```python
from build123d import *

# Parameters (mm, degrees)
F0_R     = 27
F1_DEPTH = 3
F2_R     = 27
F2_R_2   = 24
F3_DEPTH = 24
F4_R     = 1
F5_R     = 0.3


with BuildPart() as f1:
    # F0 (on Front) → F1 (new body)
    with BuildSketch(Plane.XZ):
        Circle(F0_R)
    extrude(amount=F1_DEPTH)

    # F2 (on face) → F3 (join)
    with BuildSketch(Plane(origin=(0, 0, 0), x_dir=(-1, 0, 0), z_dir=(0, 1, 0))):
        Circle(F2_R)
        Circle(F2_R_2, mode=Mode.SUBTRACT)
    extrude(amount=F3_DEPTH)

    # F4
    f4_edges = [f1.edges().sort_by_distance(p)[0] for p in [
        (-27, -3, 0),
    ]]
    fillet(f4_edges, radius=F4_R)

    # F5
    f5_edges = [f1.edges().sort_by_distance(p)[0] for p in [
        (27, 24, 0),
        (24, 24, 0),
    ]]
    fillet(f5_edges, radius=F5_R)


solid = f1.part
```
The listing builds one solid part. Answer for the finished solid, in the listing's coordinates (mm). Give positions to 0.01 mm unless a question says otherwise; leave off trailing zeros. Order: outer loops, then holes, each group sorted by start corner. A loop starts at its lowest first (then second) coordinate and runs counter-clockwise, first axis right, second up. Notation, with made-up numbers: (-14.75, 59.5) - (-1.75, 59.5) arc R35 ccw to (-1.75, 97.5) - close; hole circle Ø2 at (36.25, -33). An arc over 180 degrees is marked (long way). Use one line per item in the form item = value. Start each with the question number.
(1) A cutting plane is placed at A-A, the plane x = 0. Write down the section's boundary in (y, z).
(2) Consider line 1 (Z direction, x = 0, y = 6.25); line 2 (Y direction, x = 2, z = 7); line 3 (Z direction, x = -9, y = 18.75). Determine where each line is inside the solid, lowest interval first. Write a range as from..to.
(3) A cutting plane is placed at B-B, the plane y = 5.25. Write down the section's boundary in (x, z), then the cut area to 3 significant figures.
(4) The mould has two halves that part along X. Classify faces 1 (the flat face through (-6, 24, -24)), 2 (the cylindrical face through (23.977, 11.684, 1.055)), 3 (the flat face through (0, 0, 0)): released by +X, released by -X, zero draft, split by the parting line, or undercut.
(5) A cutting plane is placed at C-C, the plane z = 0. Write down the section's boundary in (x, y), then the cut area to 3 significant figures.
(6) Flat-ended cylindrical pins translate along their axes: pin 1 Ø12 at (x, z) = (-5.5, -1) entering from +Y; pin 2 Ø4 at (x, y) = (-8.5, 1.5) entering from -Z; pin 3 Ø3 at (y, z) = (16.5, 2.5) entering from +X. Find the tip coordinate at first contact, or state that the pin passes through.
Ans:
q1.outline = (-3, -26) arc R1 ccw to (-2, -27) - (23.7, -27) arc R0.3 ccw to (24, -26.7) - (24, -24.3) arc R0.3 ccw to (23.7, -24) - (0, -24) - (0, 24) - (23.7, 24) arc R0.3 ccw to (24, 24.3) - (24, 26.7) arc R0.3 ccw to (23.7, 27) - (-2, 27) arc R1 ccw to (-3, 26) - close
q2.line_1 = -27..-24, 24..27
q2.line_2 = -3..0
q2.line_3 = -25.46..-22.25, 22.25..25.46
q3.outline = circle Ø54 at (0, 0); hole circle Ø48 at (0, 0)
q3.area = 481 mm^2
q4.face_1 = zero draft
q4.face_2 = undercut
q4.face_3 = undercut
q5.outline = (-27, -2) arc R1 ccw to (-26, -3) - (26, -3) arc R1 ccw to (27, -2) - (27, 23.7) arc R0.3 ccw to (26.7, 24) - (24.3, 24) arc R0.3 ccw to (24, 23.7) - (24, 0) - (-24, 0) - (-24, 23.7) arc R0.3 ccw to (-24.3, 24) - (-26.7, 24) arc R0.3 ccw to (-27, 23.7) - close
q5.area = 305 mm^2
q6.pin_1 = 0
q6.pin_2 = -26.21
q6.pin_3 = 26.98
